The model under review builds one solid part; all positions refer to its coordinate system, in mm. Face numbers are marked on the shaded views. A direction names the side the tool comes from. Give positions to 0.01 mm unless a question says otherwise; leave off trailing zeros. Loops run counter-clockwise (first coordinate to the right, second up) from the corner with the lowest first, then second, coordinate; pieces in that order, holes last. Notation, with made-up numbers: (4.25, -7) - (47.25, -7) arc R23 cw to (47.25, 24) - close; hole circle Ø11 at (-24, 59). An arc over 180 degrees is marked (long way). Answer as a JSON object with one key per item and string values.
from build123d import *

# Parameters (mm, degrees)
F0_R     = 38.1
F0_R_2   = 19.05
F1_DEPTH = 7.874
F2_R     = 28.575
F2_R_2   = 19.05
F3_DEPTH = 32.766
F4_R     = 1.524


with BuildPart() as f1:
    # F0 (on Right) → F1 (new body)
    with BuildSketch(Plane.YZ):
        Circle(F0_R)
        Circle(F0_R_2, mode=Mode.SUBTRACT)
    extrude(amount=F1_DEPTH)

    # F2 (on face) → F3 (join)
    with BuildSketch(Plane.YZ.offset(7.874)):
        Circle(F2_R)
        Circle(F2_R_2, mode=Mode.SUBTRACT)
    extrude(amount=F3_DEPTH)

    # F4
    f4_edges = [f1.edges().sort_by_distance(p)[0] for p in [
        (7.874, -38.1, 0),
        (7.874, -28.575, 0),
        (40.64, -28.575, 0),
    ]]
    fillet(f4_edges, radius=F4_R)


solid = f1.part
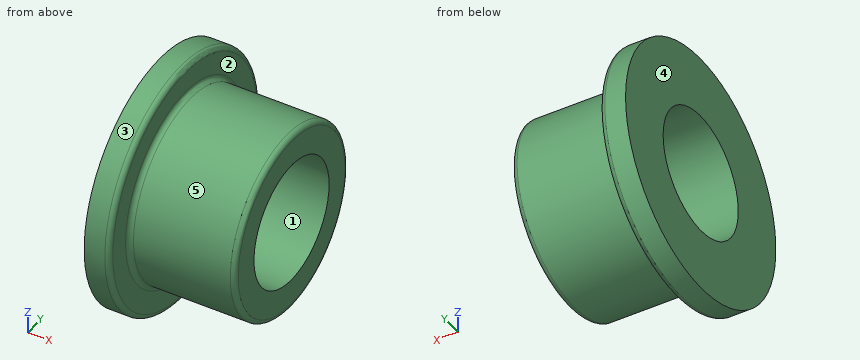
Q1. For the marked faces 4 and 5, list the 3-axis set-ups (+Z, -Z, +X, -X, +Y, -Y) from which the entire face can be reached by the end or side of a thin tool; tool diameter is ignored.
Results:
{"face 4": "+Z, -Z, -X, +Y, -Y", "face 5": "+X"}
Q2. Consider section C-C, the plane x = 4. State the section outline as (y, z) points.
Results:
{"outline": "circle Ø76.2 at (0, 0); hole circle Ø38.1 at (0, 0)"}
Q3. Consider section A-A, the plane y = 0. State the section outline as (x, z) points (3 decimals), plus the area to 3 significant figures.
Results:
{"outline": "(0, -38.1) - (6.35, -38.1) arc R1.524 ccw to (7.874, -36.576) - (7.874, -30.099) arc R1.524 cw to (9.398, -28.575) - (39.116, -28.575) arc R1.524 ccw to (40.64, -27.051) - (40.64, -19.05) - (0, -19.05) - close; (0, 19.05) - (40.64, 19.05) - (40.64, 27.051) arc R1.524 ccw to (39.116, 28.575) - (9.398, 28.575) arc R1.524 cw to (7.874, 30.099) - (7.874, 36.576) arc R1.524 ccw to (6.35, 38.1) - (0, 38.1) - close", "area": "923 mm^2"}
Q4. Clearance check with flat-ended pins moving along their axes: pin 1 Ø8 at (x, y) = (26.5, 4.5) entering from +Z; pin 2 Ø1 at (x, y) = (15.5, 18) entering from -Z; pin 3 Ø8 at (x, z) = (24.5, -26) entering from +Y. State where each tip first meets the part, or that it passes through.
Results:
{"pin 1": "stops at z = 28.57", "pin 2": "stops at z = -22.59", "pin 3": "stops at y = 18.24"}
Q5. Consider section D-D, the plane x = 22. State the section outline as (y, z) points (3 decimals), plus the area to 3 significant figures.
Results:
{"outline": "circle Ø57.15 at (0, 0); hole circle Ø38.1 at (0, 0)", "area": "1,430 mm^2"}
Q6. The part is to be moulded in two halves that separate along Z. For the marked faces 1, 2 and 3, say which applies: +Z half, -Z half, draft (parallel to the pull), parting line (faces both ways), or undercut.
Results:
{"face 1": "undercut", "face 2": "draft", "face 3": "parting line"}
Q7. To check wall thickness, follow probe 1 along Z at (x, y) = (31, 0) (3 decimals); probe 2 along Y at (x, z) = (26, 2); probe 3 along X at (y, z) = (-10, -32). State the ranges of each line that lie inside material, in increasing order. Write a range as [from, to].
Results:
{"probe 1": "z = [-28.575, -19.05], [19.05, 28.575]", "probe 2": "y = [-28.5, -18.94], [18.94, 28.5]", "probe 3": "x = [0, 7.87]"}
